Design review of the part built by this model. Coordinates are the model's own, in mm. Coordinates: 2 decimals unless noted, no trailing zeros. Write each loop counter-clockwise with the first axis right and the second up, starting at its lowest first coordinate (ties: lowest second). Pieces come first, ordered by that corner, then holes. Notation, with made-up numbers: (-18, 49) - (0, 49) arc R22 cw to (0, 82) - close; hole circle Ø4 at (81.25, 50). An arc over 180 degrees is marked (long way). Answer as a JSON object with one key per item and string values.
```python
from build123d import *

# Parameters (mm, degrees)
SKETCH_1_W             = 1.5
SKETCH_1_H             = 555.7
SM_BASE_FLANGE_1_DEPTH = 385
SKETCH_6_W             = 88.363212941
SKETCH_6_H             = 264.50252719
CUT_EXTRUDE_1_DEPTH    = 74.5
SKETCH_7_W             = 1.5
SKETCH_7_H             = 264.50252719
EXTRUDE_1_DEPTH        = 47.7
SKETCH_8_W             = 1.5
SKETCH_8_H             = 40.663212941
EXTRUDE_2_DEPTH        = 20
SKETCH_9_W             = 1.5
SKETCH_9_H             = 40.663212941
EXTRUDE_3_DEPTH        = 26
SKETCH_10_W            = 1.5
SKETCH_10_H            = 218.50252719
EXTRUDE_4_DEPTH        = 20
SKETCH_12_R            = 2.75
CUT_EXTRUDE_2_DEPTH    = 20
SKETCH_13_R            = 2.75
CUT_EXTRUDE_3_DEPTH    = 10
SKETCH_14_R            = 2.75
CUT_EXTRUDE_4_DEPTH    = 10
SKETCH_15_R            = 2.25
CUT_EXTRUDE_5_DEPTH    = 10
SKETCH_17_R            = 2.1
CUT_EXTRUDE_6_DEPTH    = 20


# Sheet-metal steps are written as plain solids
with BuildPart() as part:
    # Sketch 1 → 基体-法兰1 (new body)
    with BuildSketch(Plane.XY):
        with Locations((0.75, 277.85)):
            Rectangle(SKETCH_1_W, SKETCH_1_H)
    extrude(amount=SM_BASE_FLANGE_1_DEPTH)

    # 草图6 → 切除-拉伸1 (cut)
    with BuildSketch(Plane.ZY):
        with Locations((158.262985354, 303.520646834)):
            Rectangle(SKETCH_6_W, SKETCH_6_H)
    extrude(amount=-CUT_EXTRUDE_1_DEPTH, mode=Mode.SUBTRACT)

    # 草图7 → 凸台-拉伸1 (add)
    with BuildSketch(Plane.XY.offset(114.081378883)):
        with Locations((0.75, 303.520646834)):
            Rectangle(SKETCH_7_W, SKETCH_7_H)
    extrude(amount=EXTRUDE_1_DEPTH)

    # 草图8 → 凸台-拉伸2 (add)
    with BuildSketch(Plane.XZ.offset(-435.771910429)):
        with Locations((0.75, 182.112985353)):
            Rectangle(SKETCH_8_W, SKETCH_8_H)
    extrude(amount=EXTRUDE_2_DEPTH)

    # 草图9 → 凸台-拉伸3 (add)
    with BuildSketch(Plane(origin=(0, 171.269383239, 0), x_dir=(1, 0, 0), z_dir=(0, 1, 0))):
        with Locations((0.75, -182.112985353)):
            Rectangle(SKETCH_9_W, SKETCH_9_H)
    extrude(amount=EXTRUDE_3_DEPTH)

    # 草图10 → 凸台-拉伸4 (add)
    with BuildSketch(Plane(origin=(0, 0, 202.444591824), x_dir=(-1, 0, 0), z_dir=(0, 0, -1))):
        with Locations((-0.75, 306.520646834)):
            Rectangle(SKETCH_10_W, SKETCH_10_H)
    extrude(amount=EXTRUDE_4_DEPTH)

    # 草图12 → 切除-拉伸2 (cut)
    with BuildSketch(Plane(origin=(1.5, 0, 0), x_dir=(0, 0, -1), z_dir=(1, 0, 0))):
        with Locations((-296.5, 6.3817)):
            Circle(SKETCH_12_R)
        with Locations((-196.5, 6.3817)):
            Circle(SKETCH_12_R)
        with Locations((-96.5, 6.3817)):
            Circle(SKETCH_12_R)
    extrude(amount=-CUT_EXTRUDE_2_DEPTH, mode=Mode.SUBTRACT)

    # 草图13 → 切除-拉伸3 (cut)
    with BuildSketch(Plane(origin=(1.5, 0, 0), x_dir=(0, 0, -1), z_dir=(1, 0, 0))):
        with Locations((-377.815462169, 127.8484)):
            Circle(SKETCH_13_R)
        with Locations((-377.815462169, 277.8484)):
            Circle(SKETCH_13_R)
        with Locations((-377.815462169, 427.8484)):
            Circle(SKETCH_13_R)
    extrude(amount=-CUT_EXTRUDE_3_DEPTH, mode=Mode.SUBTRACT)

    # 草图14 → 切除-拉伸4 (cut)
    with BuildSketch(Plane(origin=(1.5, 0, 0), x_dir=(0, 0, -1), z_dir=(1, 0, 0))):
        with Locations((-296.5, 549.3183)):
            Circle(SKETCH_14_R)
        with Locations((-196.5, 549.3183)):
            Circle(SKETCH_14_R)
        with Locations((-96.5, 549.3183)):
            Circle(SKETCH_14_R)
    extrude(amount=-CUT_EXTRUDE_4_DEPTH, mode=Mode.SUBTRACT)

    # 草图15 → 切除-拉伸5 (cut)
    with BuildSketch(Plane.ZY):
        with Locations((3, 517.85)):
            Circle(SKETCH_15_R)
        with Locations((3, 437.85)):
            Circle(SKETCH_15_R)
        with Locations((3, 357.85)):
            Circle(SKETCH_15_R)
        with Locations((3, 37.85)):
            Circle(SKETCH_15_R)
        with Locations((3, 117.85)):
            Circle(SKETCH_15_R)
        with Locations((3, 197.85)):
            Circle(SKETCH_15_R)
    extrude(amount=-CUT_EXTRUDE_5_DEPTH, mode=Mode.SUBTRACT)

    # 草图17 → 切除-拉伸6 (cut)
    with BuildSketch(Plane(origin=(1.5, 0, 0), x_dir=(0, 0, -1), z_dir=(1, 0, 0))):
        with Locations((-157.14323819, 266.5334)):
            Circle(SKETCH_17_R)
        with Locations((-157.14323819, 306.5334)):
            Circle(SKETCH_17_R)
        with Locations((-157.14323819, 346.5334)):
            Circle(SKETCH_17_R)
    extrude(amount=-CUT_EXTRUDE_6_DEPTH, mode=Mode.SUBTRACT)


solid = part.part
```
(1) Take a section at A-A, the plane y = 327. Write out the cut boundary in (x, z).
Solved:
{"outline": "(0, 0) - (1.5, 0) - (1.5, 161.78) - (0, 161.78) - close; (0, 182.44) - (1.5, 182.44) - (1.5, 385) - (0, 385) - close"}
(2) Take a section at B-B, the plane z = 168.5. Write out the cut boundary in (x, y), and give its area (3 significant figures).
Solved:
{"outline": "(0, 0) - (1.5, 0) - (1.5, 197.27) - (0, 197.27) - close; (0, 415.77) - (1.5, 415.77) - (1.5, 555.7) - (0, 555.7) - close", "area": "506 mm^2"}
(3) Take a section at C-C, the plane x = 0.7. Give the number of separate pieces and of enclosed holes in the cut face, and give its area (3 significant figures).
Solved:
{"separate pieces": "1", "enclosed holes": "19", "area": "209,000 mm^2"}
(4) The part is to be moulded in two halves that separate along X. For faces 1 (the face through (0, 274, 195)), 2 (the face through (1.5, 274, 195)), say which applies: pulls with the +X half, pulls with the -X half, needs draft (parallel to the pull), parting line crosses it, or undercut.
Solved:
{"face 1": "pulls with the -X half", "face 2": "pulls with the +X half"}
(5) To check wall thickness, follow line 1 (Y direction, x = 1.2, z = 96.5); line 2 (Z direction, x = 1, y = 292); line 3 (Y direction, x = 1.1, z = 170). State the ranges of each line that lie inside material, in increasing order. Write a range as from..to.
Solved:
{"line 1": "y = 0..3.63, 9.13..546.57, 552.07..555.7", "line 2": "z = 0..161.78, 182.44..385", "line 3": "y = 0..197.27, 415.77..555.7"}
